For this review, use the dimensioned drawing (mm, ordinates from the lowest corner) and the shaded views. A direction names the side the tool comes from. Round coordinates to 2 decimals unless told otherwise and drop trailing zeros. Loops run counter-clockwise (first coordinate to the right, second up) from the corner with the lowest first, then second, coordinate; pieces in that order, holes last. Notation, with made-up numbers: (-36, 49.25) - (-31, 49.25) arc R22 ccw to (-31, 64.25) - close; hole circle Ø1 at (65, 17.25). An arc over 180 degrees is marked (long way). Answer as CSV lines item,"result". Start each with the question number.
(1) Wall thickness on L1, parallel to Y at x = 4, z = 1.25; L2, parallel to Y at x = 0.75, z = 1.8 (1 decimal); L3, parallel to Y at x = 0.5, z = 0.7 (1 decimal): over which ranges is each line inside the solid? List them lowest first.
(2) Mouldability with a two-part tool opening along Y and no side actions: class the marked faces 1, 2, 3 and 4 as released by +Y, released by -Y, zero draft, split by the parting line, or undercut.
(3) Consider section A-A (x = 4). Give the boundary of the cut face in (y, z), and give its area (3 significant figures).
(4) For P1, Ø1.3, axis at x = 2, z = 2.5, coming from the +Y side; P2, Ø1.5, axis at x = 5, z = 1, coming from the +Y side; P3, Ø2, axis at y = 22.5, z = 3, coming from the -X side, all flat-tipped, find the tip position at first contact; note any pin that passes through.
(5) Consider section B-B (z = 2.4). Give the boundary of the cut face in (x, y), and give its area (3 significant figures).
(6) Consider section D-D (y = 21.5). Give the boundary of the cut face in (x, z), and give its area (3 significant figures).
(7) For the marked faces 5 and 6, list the 3-axis set-ups (+Z, -Z, +X, -X, +Y, -Y) from which the entire face can be reached by the end or side of a thin tool; tool diameter is ignored.
(8) Consider section C-C (x = 1.5). Give the boundary of the cut face in (y, z).
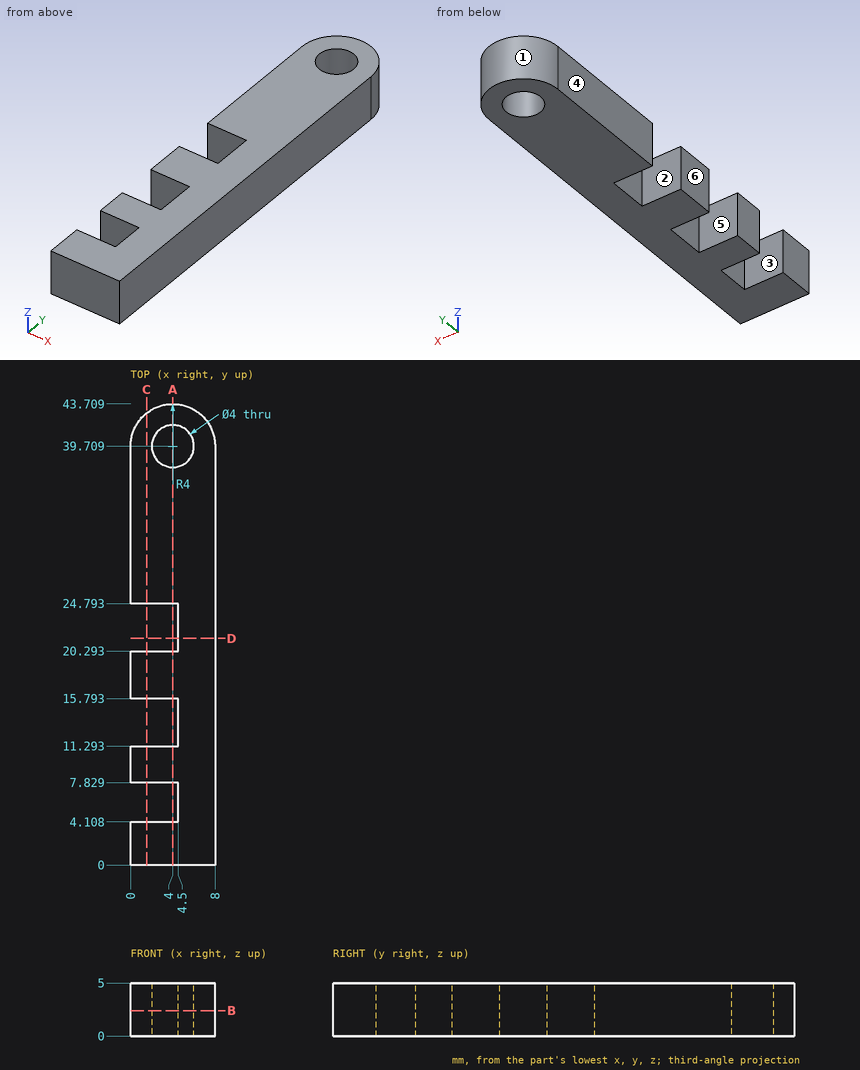
Determined:
1,L1,"y = 0 to 4.11, 7.83 to 11.29, 15.79 to 20.29, 24.79 to 37.71, 41.71 to 43.71"
1,L2,"y = 0 to 4.1, 7.8 to 11.3, 15.8 to 20.3, 24.8 to 42"
1,L3,"y = 0 to 4.1, 7.8 to 11.3, 15.8 to 20.3, 24.8 to 41.6"
2,face 1,"released by +Y"
2,face 2,"undercut"
2,face 3,"undercut"
2,face 4,"zero draft"
3,outline,"(0, 0) - (4.11, 0) - (4.11, 5) - (0, 5) - close; (7.83, 0) - (11.29, 0) - (11.29, 5) - (7.83, 5) - close; (15.79, 0) - (20.29, 0) - (20.29, 5) - (15.79, 5) - close; (24.79, 0) - (37.71, 0) - (37.71, 5) - (24.79, 5) - close; (41.71, 0) - (43.71, 0) - (43.71, 5) - (41.71, 5) - close"
3,area,"135 mm^2"
4,P1,"stops at y = 43.47"
4,P2,"stops at y = 43.7"
4,P3,"stops at x = 4.5"
5,outline,"(0, 0) - (8, 0) - (8, 39.71) arc R4 ccw to (0, 39.71) - (0, 24.79) - (4.5, 24.79) - (4.5, 20.29) - (0, 20.29) - (0, 15.79) - (4.5, 15.79) - (4.5, 11.29) - (0, 11.29) - (0, 7.83) - (4.5, 7.83) - (4.5, 4.11) - (0, 4.11) - close; hole circle Ø4 at (4, 39.71)"
5,area,"273 mm^2"
6,outline,"(4.5, 0) - (8, 0) - (8, 5) - (4.5, 5) - close"
6,area,"17.5 mm^2"
7,face 5,"+Z, -Z, -X"
7,face 6,"+Z, -Z, -X, +Y, -Y"
8,outline,"(0, 0) - (4.11, 0) - (4.11, 5) - (0, 5) - close; (7.83, 0) - (11.29, 0) - (11.29, 5) - (7.83, 5) - close; (15.79, 0) - (20.29, 0) - (20.29, 5) - (15.79, 5) - close; (24.79, 0) - (42.83, 0) - (42.83, 5) - (24.79, 5) - close"
